```python
from build123d import *

# Parameters (mm, degrees)
BOX_W        = 70.4
BOX_H        = 51
BOX_DEPTH    = 6.5
BOX003_W     = 58
BOX003_H     = 38
BOX003_DEPTH = 10
BOX001_W     = 74
BOX001_H     = 54
BOX001_DEPTH = 6.5
FILLET002_R  = 2


with BuildPart() as internal_cube:
    # Box → Box (new body)
    with BuildSketch(Plane(origin=(1.8, 1.5, 2), x_dir=(1, 0, 0), z_dir=(0, 0, 1))):
        with Locations((35.2, 25.5)):
            Rectangle(BOX_W, BOX_H)
    extrude(amount=BOX_DEPTH)


with BuildPart() as extraction_fusion:
    # Box003 → Box003 (new body)
    with BuildSketch(Plane(origin=(8, 8, -5), x_dir=(1, 0, 0), z_dir=(0, 0, 1))):
        with Locations((29, 19)):
            Rectangle(BOX003_W, BOX003_H)
    extrude(amount=BOX003_DEPTH)

    # Fusion: union internal cube
    add(internal_cube.part)


with BuildPart() as main_cube_cut:
    # Box001 → Box001 (new body)
    with BuildSketch(Plane.XY):
        with Locations((37, 27)):
            Rectangle(BOX001_W, BOX001_H)
    extrude(amount=BOX001_DEPTH)

    # Fillet002
    fillet002_edges = [main_cube_cut.edges().sort_by_distance(p)[0] for p in [
        (0, 0, 3.25),
        (0, 54, 3.25),
        (74, 0, 3.25),
        (74, 54, 3.25),
    ]]
    fillet(fillet002_edges, radius=FILLET002_R)

    # Cut: cut extraction fusion
    add(extraction_fusion.part, mode=Mode.SUBTRACT)


solid = main_cube_cut.part
```
Can you work these out from the model? Positions are in its coordinate system, mm. A direction names the side the tool comes from. Coordinates: 2 decimals unless noted, no trailing zeros. Write each loop counter-clockwise with the first axis right and the second up, starting at its lowest first coordinate (ties: lowest second). Pieces come first, ordered by that corner, then holes. Notation, with made-up numbers: M -16.5,34.5 L -3.5,34.5 A5 ccw -3.5,39.5 Z; hole C 1.5,76.25 d4. An arc over 180 degrees is marked long. Write item = value, one per line. Start each with the question number.
Q1. If we section it at B-B, the plane z = 3.5: Write out the boundary of the cut face in (x, y).
Q2. Thinking about a two-plate mould opening in X: for faces 4 (the face through (73.43, 53.4, 3.3)), 5 (the face through (37, 54, 3)), 6 (the face through (37, 52.5, 4)), which applies, released by +X, released by -X, zero draft, split by the parting line, or undercut?
Q3. On a 3-axis mill with a long thin cutter (end or side, diameter ignored), from which of +Z, -Z, +X, -X, +Y, -Y can I reach the whole of each face in a straight line? I mean faces 1 (the face through (37, 50, 2)), 2 (the face through (0.57, 0.6, 3.3)), 3 (the face through (37, 46, 1)). Say none if no direction works.
Q4. If I drill on L1, parallel to Y at x = 13.5, z = 0.5; L2, parallel to X at y = 33, z = 1.75; L3, parallel to X at y = 7, z = 5.5, over which ranges is the centre line in solid material (lowest first)? Write a range as [from, to].
Q5. If we section it at C-C, the plane x = 34: Write out the boundary of the cut face in (y, z), then the cut area to 3 significant figures.
Q6. If we section it at D-D, the plane y = 49.5: Write out the boundary of the cut face in (x, z).
Q7. If we section it at A-A, the plane y = 15: Write out the boundary of the cut face in (x, z).
Check sheet entries:
q1.outline = M 0,2 A2 ccw 2,0 L 72,0 A2 ccw 74,2 L 74,52 A2 ccw 72,54 L 2,54 A2 ccw 0,52 Z; hole M 1.8,1.5 L 72.2,1.5 L 72.2,52.5 L 1.8,52.5 Z
q2.face_4 = released by +X
q2.face_5 = zero draft
q2.face_6 = undercut
q3.face_1 = +Z
q3.face_2 = +Z, -Z, -X, -Y
q3.face_3 = +Z, -Z
q4.L1 = [0, 8], [46, 54]
q4.L2 = [0, 8], [66, 74]
q4.L3 = [0, 1.8], [72.2, 74]
q5.outline = M 0,0 L 8,0 L 8,2 L 1.5,2 L 1.5,6.5 L 0,6.5 Z; M 46,0 L 54,0 L 54,6.5 L 52.5,6.5 L 52.5,2 L 46,2 Z
q5.area = 45.5 mm²
q6.outline = M 0,0 L 74,0 L 74,6.5 L 72.2,6.5 L 72.2,2 L 1.8,2 L 1.8,6.5 L 0,6.5 Z
q7.outline = M 0,0 L 8,0 L 8,2 L 1.8,2 L 1.8,6.5 L 0,6.5 Z; M 66,0 L 74,0 L 74,6.5 L 72.2,6.5 L 72.2,2 L 66,2 Z
